Design review of the part built by this model. Coordinates are the model's own, in mm. A direction names the side the tool comes from. Round coordinates to 2 decimals unless told otherwise and drop trailing zeros. Loops run counter-clockwise (first coordinate to the right, second up) from the corner with the lowest first, then second, coordinate; pieces in that order, holes last. Notation, with made-up numbers: (-5, -34) -> (26, -34) arc R20 ccw to (26, -12) -> close; hole circle Ø7 at (14, 20.5). An arc over 180 degrees is marked (long way). Answer as CSV lines item,"result". Start each with the question number.
(1) Machinability: for faces 1 (the face through (-40, 13, 4)), 2 (the face through (-18, 0, 25)), 3 (the face through (-78, 8.3, 17)), 4 (the face through (-69, 12, -1)), which of the approach directions +Z, -Z, +X, -X, +Y, -Y give a long, thin tool a straight path to every point of the face, cutting with its end or side? Answer none if there is none.
(2) Take a section at A-A, the plane x = 18. Write out the cut boundary in (y, z), and give its area (4 significant figures).
(3) Take a section at B-B, the plane y = 157. Write out the cut boundary in (x, z), and give its area (3 significant figures).
(4) Draft analysis for pull direction Z (two halves, no side actions). For faces 5 (the face through (57, 13, 28)), 6 (the face through (-10, 129, 24)), 7 (the face through (28, 21, 3)), state which applies: +Z half, -Z half, draft (parallel to the pull), parting line (faces both ways), or undercut.
(5) Take a section at C-C, the plane z = 13. State how many separate pieces and enclosed holes the cut face has, and give its area (3 significant figures).
(6) Take a section at D-D, the plane x = -60. Write out the cut boundary in (y, z), and give its area (3 significant figures).
(7) For P1, Ø3, axis at y = 109, z = 21, coming from the +X side; P2, Ø1.9, axis at y = 12.5, z = 19, coming from the +X side; P3, Ø1.6, axis at x = -76.5, y = 13, coming from the +Z side; P4, Ø2, axis at x = -12, y = 32, coming from the +Z side, all flat-tipped, find the tip position at first contact; note any pin that passes through.
(8) To check wall thickness, follow line 1 (Y direction, x = -86.75, z = 9); line 2 (Y direction, x = -77.5, z = 10.5); line 3 (Y direction, x = -34, z = -21). State the ranges of each line that lie inside material, in increasing order. Write a range as from..to.
from build123d import *

# Parameters (mm, degrees)
SKETCH1_W                  = 151
SKETCH1_H                  = 58
SKETCH1_W_2                = 76
SKETCH1_H_2                = 38
BOSS_EXTRUDE1_DEPTH        = 25
SKETCH2_W                  = 76
SKETCH2_H                  = 10
CUT_EXTRUDE1_DEPTH         = 2
SKETCH3_W                  = 40
SKETCH3_H                  = 10
CUT_EXTRUDE2_DEPTH         = 2
SKETCH4_W                  = 76
SKETCH4_H                  = 7.5
BOSS_EXTRUDE2_DEPTH        = 5
SKETCH6_W                  = 20
SKETCH6_H                  = 10
BOSS_EXTRUDE3_DEPTH        = 210
SKETCH7_W                  = 10
SKETCH7_H                  = 7.5
BOSS_EXTRUDE4_DEPTH        = 33
BOSS_EXTRUDE5_DEPTH        = 5
FILLET2_R                  = 2
M2_5_CLEARANCE_HOLE1_D     = 3.1
M2_5_CLEARANCE_HOLE1_DEPTH = 16.068666041
M2_5_CLEARANCE_HOLE1_TIP   = 0.931333959
M2_5_CLEARANCE_HOLE2_D     = 3.1
M2_5_CLEARANCE_HOLE2_DEPTH = 16.068666041
M2_5_CLEARANCE_HOLE2_TIP   = 0.931333959
SKETCH19_W                 = 5
SKETCH19_H                 = 8
SKETCH19_W_2               = 5.4
SKETCH19_H_2               = 8.4
CUT_EXTRUDE4_DEPTH         = 25.2
SKETCH25_W                 = 47
SKETCH25_H                 = 28
SKETCH25_W_2               = 14
CUT_EXTRUDE5_DEPTH         = 255.02755756
FILLET3_R                  = 5


with BuildPart() as part:
    # Sketch1 → Boss-Extrude1 (new body)
    with BuildSketch(Plane(origin=(0, 0, 0), x_dir=(1, 0, 0), z_dir=(0, 1, 0))):
        with Locations((-16.5, 0)):
            Rectangle(SKETCH1_W, SKETCH1_H)
        with Locations((0, -5)):
            Rectangle(SKETCH1_W_2, SKETCH1_H_2, mode=Mode.SUBTRACT)
    extrude(amount=BOSS_EXTRUDE1_DEPTH)

    # Sketch2 → Cut-Extrude1 (cut)
    with BuildSketch(Plane.XY.offset(-14)):
        with Locations((0, 12.5)):
            Rectangle(SKETCH2_W, SKETCH2_H)
    extrude(amount=-CUT_EXTRUDE1_DEPTH, mode=Mode.SUBTRACT)

    # Sketch3 → Cut-Extrude2 (cut)
    with BuildSketch(Plane(origin=(-38, 0, 0), x_dir=(0, 0, -1), z_dir=(1, 0, 0))):
        with Locations((-4, 12.5)):
            Rectangle(SKETCH3_W, SKETCH3_H)
    cut_extrude2 = extrude(amount=-CUT_EXTRUDE2_DEPTH, mode=Mode.SUBTRACT)

    # Mirror1: Cut-Extrude2 across plane
    add(cut_extrude2.mirror(Plane(origin=(0, 0, 0), x_dir=(0, 0, 1), z_dir=(1, 0, 0))), mode=Mode.SUBTRACT)

    # Sketch4 → Boss-Extrude2 (add)
    with BuildSketch(Plane(origin=(0, 0, 24), x_dir=(-1, 0, 0), z_dir=(0, 0, -1))):
        with Locations((0, 21.25)):
            Rectangle(SKETCH4_W, SKETCH4_H)
    extrude(amount=BOSS_EXTRUDE2_DEPTH)

    # Sketch6 → Boss-Extrude3 (add)
    with BuildSketch(Plane(origin=(0, 25, 0), x_dir=(1, 0, 0), z_dir=(0, 1, 0))):
        with Locations((0, -24)):
            Rectangle(SKETCH6_W, SKETCH6_H)
    extrude(amount=BOSS_EXTRUDE3_DEPTH)

    # Sketch7 → Boss-Extrude4 (add)
    with BuildSketch(Plane(origin=(0, 0, 19), x_dir=(-1, 0, 0), z_dir=(0, 0, -1))):
        with Locations((-33, 21.25)):
            Rectangle(SKETCH7_W, SKETCH7_H)
        with Locations((33, 21.25)):
            Rectangle(SKETCH7_W, SKETCH7_H)
    extrude(amount=BOSS_EXTRUDE4_DEPTH)

    # Sketch8 → Boss-Extrude5 (add, symmetric)
    with BuildSketch(Plane(origin=(0, 0, 0), x_dir=(0, 0, -1), z_dir=(1, 0, 0))):
        Polygon((-19, 134.090909091), (29, 25), (14, 25), (-19, 100), align=None)
    extrude(amount=BOSS_EXTRUDE5_DEPTH, both=True)

    # Fillet2
    fillet2_edges = [part.edges().sort_by_distance(p)[0] for p in [
        (-5, 62.5, 2.5),
        (-5, 79.545454545, -5),
        (5, 62.5, 2.5),
        (5, 79.545454545, -5),
        (10, 130, 29),
        (10, 130, 19),
        (-10, 130, 19),
        (-10, 130, 29),
    ]]
    fillet(fillet2_edges, radius=FILLET2_R)

    # M2.5 Clearance Hole1
    with Locations(Plane(origin=(59, 0, 0), x_dir=(0, 0, -1), z_dir=(1, 0, 0))):
        with Locations((-19, 12.5), (-9, 12.5)):
            Hole(M2_5_CLEARANCE_HOLE1_D / 2, depth=M2_5_CLEARANCE_HOLE1_DEPTH)
            with Locations((0, 0, -(M2_5_CLEARANCE_HOLE1_DEPTH + M2_5_CLEARANCE_HOLE1_TIP / 2))):  # 118° drill point
                Cone(0, M2_5_CLEARANCE_HOLE1_D / 2, M2_5_CLEARANCE_HOLE1_TIP, mode=Mode.SUBTRACT)

    # M2.5 Clearance Hole2
    with Locations(Plane.ZY.offset(92)):
        with Locations((9, 12.5), (19, 12.5)):
            Hole(M2_5_CLEARANCE_HOLE2_D / 2, depth=M2_5_CLEARANCE_HOLE2_DEPTH)
            with Locations((0, 0, -(M2_5_CLEARANCE_HOLE2_DEPTH + M2_5_CLEARANCE_HOLE2_TIP / 2))):  # 118° drill point
                Cone(0, M2_5_CLEARANCE_HOLE2_D / 2, M2_5_CLEARANCE_HOLE2_TIP, mode=Mode.SUBTRACT)

    # Sketch19 → Cut-Extrude4 (cut)
    with BuildSketch(Plane.XY.offset(29)):
        with Locations((44.5, 12.5)):
            Rectangle(SKETCH19_W, SKETCH19_H)
        with Locations((44.5, 12.5)):
            Rectangle(SKETCH19_W_2, SKETCH19_H_2)
        with Locations((-77.5, 12.5)):
            Rectangle(SKETCH19_W_2, SKETCH19_H_2)
    extrude(amount=-CUT_EXTRUDE4_DEPTH, mode=Mode.SUBTRACT)

    # Sketch25 → Cut-Extrude5 (cut, through all)
    with BuildSketch(Plane.XZ):
        with Locations((-68.5, -15)):
            Rectangle(SKETCH25_W, SKETCH25_H)
        with Locations((52, -15)):
            Rectangle(SKETCH25_W_2, SKETCH25_H)
    extrude(amount=-CUT_EXTRUDE5_DEPTH, mode=Mode.SUBTRACT)

    # Fillet3
    fillet3_edges = [part.edges().sort_by_distance(p)[0] for p in [
        (-92, 12.5, -1),
        (45, 12.5, -29),
        (-45, 12.5, -1),
        (-45, 12.5, -29),
        (45, 12.5, -1),
        (59, 12.5, -1),
        (59, 12.5, 29),
        (-92, 12.5, 29),
    ]]
    fillet(fillet3_edges, radius=FILLET3_R)


solid = part.part
The answers:
1,face 1,"none"
1,face 2,"+Z, -Z, +X, -X, -Y"
1,face 3,"+Z"
1,face 4,"-Z, -X, +Y, -Y"
2,outline,"(0, -29) -> (25, -29) -> (25, -14) -> (17.5, -14) -> (17.5, -16) -> (7.5, -16) -> (7.5, -14) -> (0, -14) -> close; (0, 24) -> (17.5, 24) -> (17.5, 19) -> (25, 19) -> (25, 29) -> (0, 29) -> close"
2,area,"517.5 mm²"
3,outline,"(-10, 21) arc R2 ccw to (-8, 19) -> (8, 19) arc R2 ccw to (10, 21) -> (10, 27) arc R2 ccw to (8, 29) -> (-8, 29) arc R2 ccw to (-10, 27) -> close"
3,area,"197 mm²"
4,face 5,"+Z half"
4,face 6,"draft"
4,face 7,"undercut"
5,separate pieces,"3"
5,enclosed holes,"2"
5,area,"2,230 mm²"
6,outline,"(0, -1) -> (25, -1) -> (25, 29) -> (0, 29) -> close"
6,area,"750 mm²"
7,P1,"x = 10"
7,P2,"x = 41.8"
7,P3,"z = 3.8"
7,P4,"through"
8,line 1,"0..10.95, 14.05..25"
8,line 2,"0..8.3, 16.7..25"
8,line 3,"0..25"
